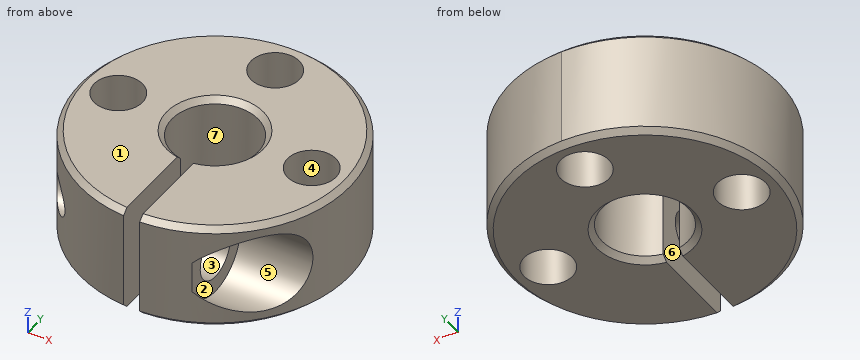
Autodesk Inventor part; units mm, degrees
ref_plane "to_bolt_XY" through (5, -8, 0) normal (1, 0, 0) x (0, 0, -1)
ref_plane "to_bolt_YZ" through (5, -8, 0) normal (0, 0, -1) x (0, 1, 0)
ref_plane "to_bolt_ZX" through (5, -8, 0) normal (0, 1, 0) x (1, 0, 0)
sketch "Sketch_14" plane through (0, 0, 0) normal (1, 0, 0) x (0, 1, 0)
  line L0 (0, -5) -> (0, 5)
  line L1 (0, 5) -> (12, 5)
  line L2 (12, 5) -> (12.5, 4.5)
  line L3 (12.5, 4.5) -> (12.5, -4.5)
  line L4 (12.5, -4.5) -> (12, -5)
  line L5 (12, -5) -> (0, -5)
  line L6 (0, -5) -> (0, 5)
revolve "Revolution1" add sketch "Sketch_14" angle 360 about axis through (0, 0, -5) along (0, 0, -1)
sketch "Sketch_15" plane through (0, 0, 0) normal (1, 0, 0) x (0, 1, 0)
  line L0 (0, -5) -> (0, 5)
  line L1 (0, 5) -> (4.5, 5)
  line L2 (4.5, 5) -> (4, 4.5)
  line L3 (4, 4.5) -> (4, -4.5)
  line L4 (4, -4.5) -> (4.5, -5)
  line L5 (4.5, -5) -> (0, -5)
  line L6 (0, -5) -> (0, 5)
revolve "Revolution2" cut sketch "Sketch_15" angle 360 about axis through (0, 0, -5) along (0, 0, -1)
sketch "Sketch_16" plane through (0, 0, 0) normal (0, 0, 1) x (1, 0, 0)
  arc A0 (-0.75, -13.4792) -> (0.75, -13.4792) centre (0, 0) ccw
  line L0 (0.75, -13.4792) -> (0.75, 0)
  line L1 (0.75, 0) -> (-0.75, 0)
  line L2 (-0.75, 0) -> (-0.75, -13.4792)
extrude "Extrusion1" cut sketch "Sketch_16" along normal mid plane 10
sketch "Sketch4" plane through (0, 0, -5) normal (0, 0, -1) x (-1, 0, 0)
  point P0 (-9, 0)
hole "Hole1" at (9, 0, -5) direction (0, 0, 1) diameter 4.5 depth 10
sketch "Sketch5" plane through (0, 0, -5) normal (0, 0, -1) x (-1, 0, 0)
  point P0 (9, 0)
hole "Hole2" at (-9, 0, -5) direction (0, 0, 1) diameter 4.5 depth 10
sketch "Sketch6" plane through (0, 0, -5) normal (0, 0, -1) x (-1, 0, 0)
  point P0 (0, 9)
hole "Hole3" at (0, 9, -5) direction (0, 0, 1) diameter 4.5 depth 10
sketch "Sketch_23" plane through (0, -8, 0) normal (0, 1, 0) x (1, 0, 0)
  line L0 (12.5, 0) -> (0, 0)
  line L1 (0, 0) -> (0, 2.25)
  line L2 (0, 2.25) -> (5, 2.25)
  line L3 (5, 2.25) -> (5, 3.75)
  line L4 (5, 3.75) -> (12.5, 3.75)
  line L5 (12.5, 3.75) -> (12.5, 0)
  line L6 (12.5, 0) -> (0, 0)
revolve "Revolution3" cut sketch "Sketch_23" angle 360 about axis through (12.5, -8, 0) along (1, 0, 0)
sketch "Sketch8" plane through (-0.75, -11.9765, 5) normal (1, 0, 0) x (0, 0, -1)
  point P0 (5, 3.9765)
hole "Hole4" at (-0.75, -8, 0) direction (-1, 0, 0) diameter 3.242 depth 10.2159 countersink diameter 4 countersink angle 90
ref_plane "to_bolt_XY" through (5, -8, 0) normal (1, 0, 0) x (0, 0, -1)
ref_plane "to_bolt_YZ" through (5, -8, 0) normal (0, 0, -1) x (0, 1, 0)
ref_plane "to_bolt_ZX" through (5, -8, 0) normal (0, 1, 0) x (1, 0, 0)
properties part number "SCST8-10b"
The listing builds one solid part. Answer for the finished solid, in the listing's coordinates (mm). Face numbers are marked on the shaded views. A direction names the side the tool comes from. Round coordinates to 2 decimals unless told otherwise and drop trailing zeros. Order: outer loops, then holes, each group sorted by start corner. A loop starts at its lowest first (then second) coordinate and runs counter-clockwise, first axis right, second up. Notation, with made-up numbers: (85, 25) -> (97, 25) arc R26 ccw to (97, 42) -> close; hole circle Ø5 at (65.5, -19.75). An arc over 180 degrees is marked (long way). One line per item, written item: value.
Item 1: Find section A-A, the plane y = 0. Give the vertices of the cut face in (x, z).
Taken from the geometry:
outline: (-12.5, -4.5) -> (-12, -5) -> (-11.25, -5) -> (-11.25, 5) -> (-12, 5) -> (-12.5, 4.5) -> close; (-6.75, -5) -> (-4.5, -5) -> (-4, -4.5) -> (-4, 4.5) -> (-4.5, 5) -> (-6.75, 5) -> close; (4, -4.5) -> (4.5, -5) -> (6.75, -5) -> (6.75, 5) -> (4.5, 5) -> (4, 4.5) -> close; (11.25, -5) -> (12, -5) -> (12.5, -4.5) -> (12.5, 4.5) -> (12, 5) -> (11.25, 5) -> close
Item 2: Given P1, Ø3, axis at y = 5.5, z = -4, coming from the -X side; P2, Ø1.5, axis at y = -7.5, z = -3, coming from the -X side; P3, Ø3.5, axis at y = -9, z = -1, coming from the +X side, each flat-ended and moving along its own axis, determine where each tip first touches the part or whether it passes through.
Taken from the geometry:
P1: stops at x = -11.84
P2: stops at x = -10.52
P3: stops at x = 5
Item 3: Find section B-B, the plane z = 3. Give the vertices of the cut face in (x, y), then the cut area to 3 significant figures.
Taken from the geometry:
outline: (-0.75, -12.48) -> (-0.75, -3.93) arc R4 cw (long way) to (0.75, -3.93) -> (0.75, -12.48) arc R12.5 ccw to (7.15, -10.25) -> (5, -10.25) -> (5, -5.75) -> (11.1, -5.75) arc R12.5 ccw (long way) to start; hole circle Ø4.5 at (-9, 0); hole circle Ø4.5 at (0, 9); hole circle Ø4.5 at (9, 0)
area: 360 mm2
Item 4: Find section C-C, the plane x = -3.25. State how many separate pieces and enclosed holes the cut face has, then the cut area to 3 significant figures.
Taken from the geometry:
separate pieces: 2
enclosed holes: 1
area: 185 mm2
Item 5: Straight lines are drawn through the part: L1, parallel to X at y = 0, z = 2.75; L2, parallel to Y at x = 0, z = -2; L3, parallel to Y at x = -10, z = 1.25. For each, find the intervals that lie inside material, in ascending order.
Taken from the geometry:
L1: x = -12.5 to -11.25, -6.75 to -4, 4 to 6.75, 11.25 to 12.5
L2: y = 4 to 6.75, 11.25 to 12.5
L3: y = -6.97 to -2.02, 2.02 to 7.5
Item 6: For the marked faces 5, 6 and 7, determine the directions among +Z, -Z, +X, -X, +Y, -Y from which every point of the face is accessible in a straight line to the end or side of a thin tool.
Taken from the geometry:
face 5: +X
face 6: +Z, -Z, -Y
face 7: +Z, -Z
Item 7: For a pull along Z with two mould halves and no side action, classify the marked faces 1, 2, 3 and 4 as released by +Z, released by -Z, zero draft, split by the parting line, or undercut.
Taken from the geometry:
face 1: released by +Z
face 2: undercut
face 3: undercut
face 4: zero draft
